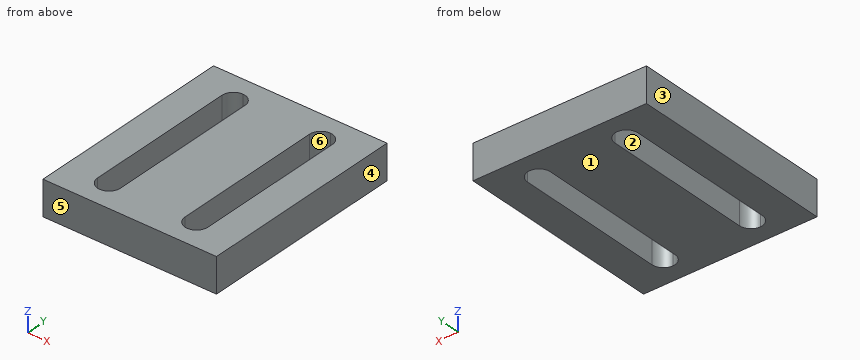
Autodesk Inventor part; units mm, degrees
ref_plane "YZ Plane" through (0, 0, 0) normal (1, 0, 0) x (0, 1, 0)
ref_plane "XZ Plane" through (0, 0, 0) normal (0, 1, 0) x (-1, 0, 0)
ref_plane "XY Plane" through (0, 0, 0) normal (0, 0, 1) x (1, 0, 0)
sketch "Skizze3" plane through (0, 0, 0) normal (0, 0, 1) x (1, 0, 0)
  line L0 (0, 0) -> (50, 0)
  line L1 (0, 0) -> (50, 0)
  line L2 (50, 0) -> (50, -60)
  line L3 (50, -60) -> (0, -60)
  line L4 (0, -60) -> (0, 0)
  line L5 (40.9, -4.8) -> (34.3, -4.8)
  line L6 (34.3, -4.8) -> (34.3, -55.2)
  line L7 (34.3, -55.2) -> (40.9, -55.2)
  line L8 (40.9, -55.2) -> (40.9, -4.8)
  line L9 (9.1, -4.8) -> (15.7, -4.8)
  line L10 (15.7, -4.8) -> (15.7, -55.2)
  line L11 (15.7, -55.2) -> (9.1, -55.2)
  line L12 (9.1, -55.2) -> (9.1, -4.8)
  dimension "d20" = 50
  dimension "d21" = 60
  dimension "d27" = 6.6
  dimension "d28" = 6.6
extrude "Extrusion6" add sketch "Skizze3" along normal blind 10
fillet "Rundung5" radius 3.3 8 edges at (34.3, -4.8, 5) (9.1, -4.8, 5) (40.9, -4.8, 5) (15.7, -4.8, 5) (34.3, -55.2, 5) (9.1, -55.2, 5) (40.9, -55.2, 5) (15.7, -55.2, 5)
properties part number "Fuß Steher"
Geometry check sheet. Reference: the model listing, model coordinates, mm. Face numbers are marked on the shaded views. A direction names the side the tool comes from. Give positions to 0.01 mm unless a question says otherwise; leave off trailing zeros. Loops run counter-clockwise (first coordinate to the right, second up) from the corner with the lowest first, then second, coordinate; pieces in that order, holes last. Notation, with made-up numbers: (44.5, 17.25) -> (86.5, 17.25) arc R22 ccw to (86.5, 38.25) -> close; hole circle Ø9 at (9, 28.25). An arc over 180 degrees is marked (long way). Answer in a Markdown table with one row per item. Add a question column.
1) Cross-section at C-C on x = 13.5. Record the boundary of the cut face in (y, z).
2) Cross-section at A-A on y = -26. Record the boundary of the cut face in (x, z), and give its area (3 significant figures).
3) Draft check along X on the marked faces 3, 4, 5 and 6. Enter one of: pulls with the +X half, pulls with the -X half, needs draft (parallel to the pull), parting line crosses it, or undercut.
4) Gauge pin test, flat end, axial feed: P1, Ø2, axis at x = 28, z = 7, coming from the +Y side. Record the tip position at first contact, or that the pin passes through.
5) Material ranges on probe 1 along X at (y, z) = (-27.5, 8.75); probe 2 along X at (y, z) = (-54, 5.75); probe 3 along Y at (x, z) = (11, 4.5), recorded low to high. Write a range as from..to.
6) Cross-section at B-B on z = 8. State how many separate pieces and enclosed holes the cut face has, and give its area (3 significant figures).
7) Cross-section at D-D on y = -7. Record the boundary of the cut face in (x, z), and give its area (3 significant figures).
8) Set-up check for the marked faces 1 and 2: record each of +Z, -Z, +X, -X, +Y, -Y from which the full face is reachable in a straight line by a thin tool's end or side.
Outcome:
| question | item | result |
|---|---|---|
| 1 | outline | (-60, 0) -> (-55.01, 0) -> (-55.01, 10) -> (-60, 10) -> close; (-4.99, 0) -> (0, 0) -> (0, 10) -> (-4.99, 10) -> close |
| 2 | outline | (0, 0) -> (9.1, 0) -> (9.1, 10) -> (0, 10) -> close; (15.7, 0) -> (34.3, 0) -> (34.3, 10) -> (15.7, 10) -> close; (40.9, 0) -> (50, 0) -> (50, 10) -> (40.9, 10) -> close |
| 2 | area | 368 mm^2 |
| 3 | face 3 | pulls with the -X half |
| 3 | face 4 | pulls with the +X half |
| 3 | face 5 | needs draft |
| 3 | face 6 | undercut |
| 4 | P1 | stops at y = 0 |
| 5 | probe 1 | x = 0..9.1, 15.7..34.3, 40.9..50 |
| 5 | probe 2 | x = 0..9.85, 14.95..35.05, 40.15..50 |
| 5 | probe 3 | y = -60..-54.89, -5.11..0 |
| 6 | separate pieces | 1 |
| 6 | enclosed holes | 2 |
| 6 | area | 2,350 mm^2 |
| 7 | outline | (0, 0) -> (9.29, 0) -> (9.29, 10) -> (0, 10) -> close; (15.51, 0) -> (34.49, 0) -> (34.49, 10) -> (15.51, 10) -> close; (40.71, 0) -> (50, 0) -> (50, 10) -> (40.71, 10) -> close |
| 7 | area | 376 mm^2 |
| 8 | face 1 | -Z, +X, -X, +Y, -Y |
| 8 | face 2 | +Z, -Z |
